Here's the drawing with two shaded views (mm, measured from the low corner). I have some questions. Give positions to 0.01 mm unless a question says otherwise; leave off trailing zeros. Write each loop counter-clockwise with the first axis right and the second up, starting at its lowest first coordinate (ties: lowest second). Pieces come first, ordered by that corner, then holes. Notation, with made-up numbers: (21, 3.5) - (44, 3.5) arc R23 cw to (44, 39.5) - close; hole circle Ø1 at (89.25, 13). An arc over 180 degrees is marked (long way). Use one line per item in the form item = value.
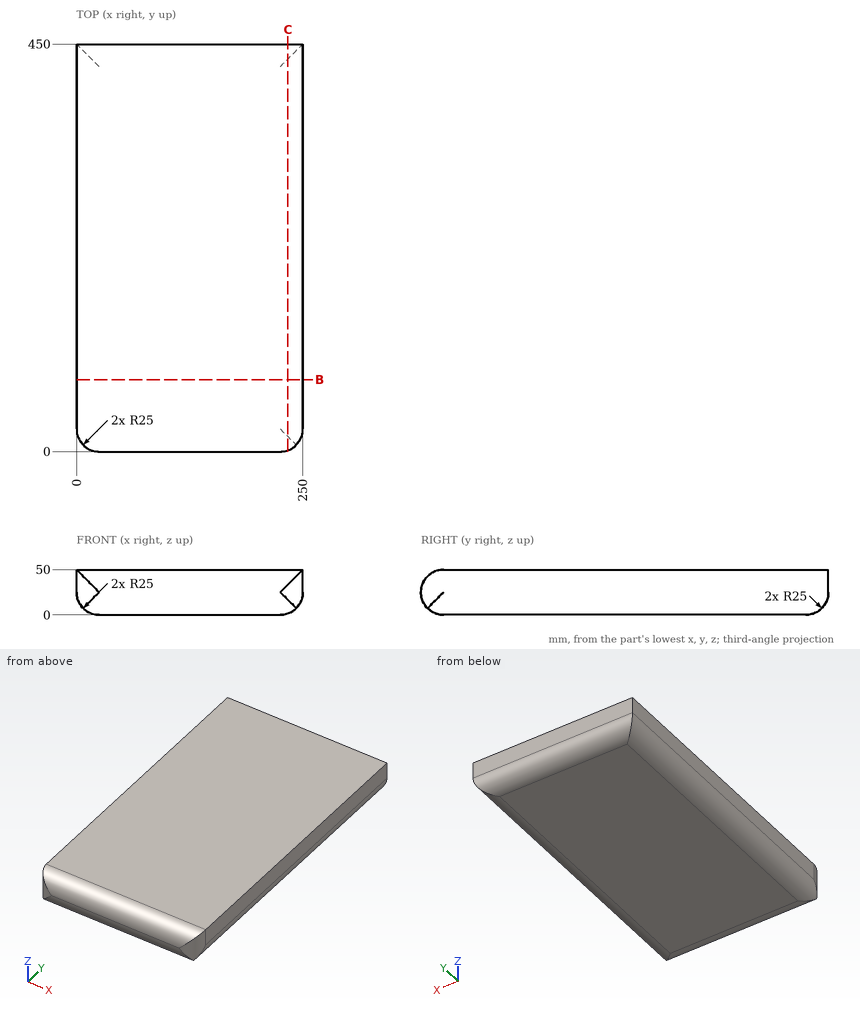
1. Imagine slicing it at C-C, the plane x = 233.5. List the corners of the cut face in (y, z) for me.
Response values:
outline = (1.49, 16.5) arc R25 ccw to (16.5, 1.49) - (433.5, 1.49) arc R25 ccw to (450, 25) - (450, 50) - (25, 50) arc R25 ccw to (1.49, 33.5) - close
2. If I drill on line 1 (X direction, y = 162, z = 24.5) (3 decimals); line 2 (X direction, y = 22, z = 20); line 3 (Y direction, x = 108, z = 28), over which ranges is the centre line in solid material (lowest first)? Write a range as from..to.
Response values:
line_1 = 0.005..249.995
line_2 = 0.51..249.49
line_3 = 0.18..450
3. Imagine slicing it at B-B, the plane y = 79.5. List the corners of the cut face in (x, z) for me, and give its area (3 significant figures).
Response values:
outline = (0, 25) arc R25 ccw to (25, 0) - (225, 0) arc R25 ccw to (250, 25) - (250, 50) - (0, 50) - close
area = 12,200 mm²
4. For pin 1 (6 mm diameter, centred on x = 157.5, z = 21.5, fed in from +Y) (3 decimals); pin 2 (10 mm diameter, centred on x = 77.5, z = 32, fed in from -Y); pin 3 (6 mm diameter, centred on x = 143, z = 5.5, fed in from +Y), each with a flat end and sliding along its axis, tell me the tip position at first contact or that it passes through.
Response values:
pin_1 = 449.995
pin_2 = 0.08
pin_3 = 443.78
